Geometry check sheet. Reference: the model listing, model coordinates, mm. Face numbers are marked on the shaded views. A direction names the side the tool comes from. Round coordinates to 2 decimals unless told otherwise and drop trailing zeros. Write each loop counter-clockwise with the first axis right and the second up, starting at its lowest first coordinate (ties: lowest second). Pieces come first, ordered by that corner, then holes. Notation, with made-up numbers: M 11,77.5 L 15,77.5 A26 cw 15,92.5 Z; hole C 57.5,35.5 d3. An arc over 180 degrees is marked long. Answer in a Markdown table with one row per item. Add a question column.
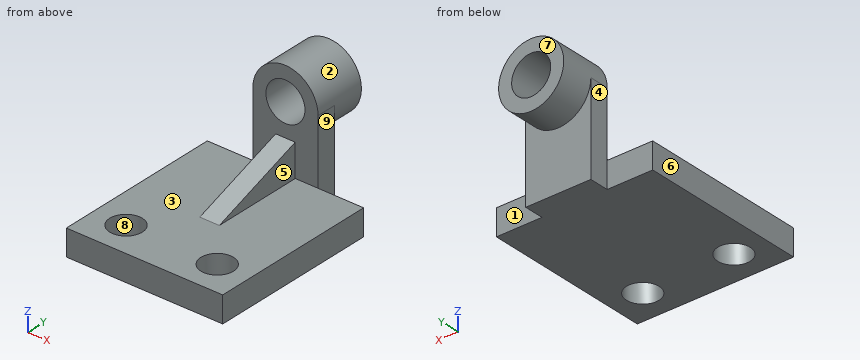
from build123d import *

# Parameters (mm, degrees)
SKETCH_1_W                  = 120
SKETCH_1_H                  = 130
EXTRUDE_1_DEPTH             = 20
SKETCH_2_R                  = 12.5
CUT_EXTRUDE_1_DEPTH         = 91.691785736
SKETCH_3_W                  = 50
SKETCH_3_H                  = 70
EXTRUDE_2_DEPTH             = 15
SKETCH_4_R                  = 25
EXTRUDE_3_DEPTH             = 25
EXTRUDE_3_DIRECTION_2_REACH = 173.828
SKETCH_5_R                  = 15
CUT_EXTRUDE_2_DEPTH         = 204.776838723
RIB_1_REACH                 = 155.786
SKETCH_6_WALL_W             = 383.901473722
SKETCH_6_WALL_H             = 15


with BuildPart() as part:
    # Эскиз1 → Бобышка-Вытянуть1 (new body)
    with BuildSketch(Plane.XY):
        Rectangle(SKETCH_1_W, SKETCH_1_H)
    extrude(amount=EXTRUDE_1_DEPTH)

    # Эскиз2 → Вырез-Вытянуть1 (cut, through all)
    with BuildSketch(Plane.XY.offset(20)):
        with Locations((35, -40)):
            Circle(SKETCH_2_R)
    cut_extrude_1 = extrude(amount=-CUT_EXTRUDE_1_DEPTH, mode=Mode.SUBTRACT)

    # Зеркальное отражение1: Вырез-Вытянуть1 across plane
    add(cut_extrude_1.mirror(Plane(origin=(0, 0, 0), x_dir=(0, 0, 1), z_dir=(1, 0, 0))), mode=Mode.SUBTRACT)

    # Эскиз3 → Бобышка-Вытянуть2 (add)
    with BuildSketch(Plane(origin=(0, 65, 0), x_dir=(1, 0, 0), z_dir=(0, 1, 0))):
        with Locations((0, -35)):
            Rectangle(SKETCH_3_W, SKETCH_3_H)
    extrude(amount=EXTRUDE_2_DEPTH)

    # Эскиз4 → Бобышка-Вытянуть3 (add)
    with BuildSketch(Plane(origin=(0, 80, 0), x_dir=(1, 0, 0), z_dir=(0, 1, 0))):
        with Locations(Location((0, -70, 0), (0, 0, 270))):
            Circle(SKETCH_4_R)
    extrude(amount=EXTRUDE_3_DEPTH)

    # Бобышка-Вытянуть3 direction 2: up to this face of the body (flat: up to its plane)
    extrude_3_direction_2_end = Plane(part.part.faces().sort_by_distance((0, 65, 45))[0])
    # Эскиз4 → Бобышка-Вытянуть3 direction 2 (add, up to the picked face)
    with BuildSketch(Plane(origin=(0, 80, 0), x_dir=(1, 0, 0), z_dir=(0, 1, 0)), mode=Mode.PRIVATE) as extrude_3_direction_2_sk1:
        with Locations(Location((0, -70, 0), (0, 0, 270))):
            Circle(SKETCH_4_R)
    extrude_3_direction_2_tool1 = split(extrude(extrude_3_direction_2_sk1.sketch, amount=-EXTRUDE_3_DIRECTION_2_REACH, mode=Mode.PRIVATE), bisect_by=extrude_3_direction_2_end, keep=Keep.BOTH, mode=Mode.PRIVATE)
    add(extrude_3_direction_2_tool1.solids().sort_by(Axis((0, 80, 70), (0, -1, 0)))[0])

    # Эскиз5 → Вырез-Вытянуть2 (cut, through all)
    with BuildSketch(Plane(origin=(0, 105, 0), x_dir=(1, 0, 0), z_dir=(0, 1, 0))):
        with Locations(Location((0, -70, 0), (0, 0, 270))):
            Circle(SKETCH_5_R)
    extrude(amount=-CUT_EXTRUDE_2_DEPTH, mode=Mode.SUBTRACT)

    # Эскиз6 wall → Ребро1 (add, up to next)
    with BuildSketch(Plane(origin=(0, 30, 32.5), x_dir=(0, -0.941741911595, -0.336336396998), z_dir=(0, 0.336336396998, -0.941741911595)), mode=Mode.PRIVATE) as rib_1_sk1:
        Rectangle(SKETCH_6_WALL_W, SKETCH_6_WALL_H)
    rib_1_tool1 = extrude(rib_1_sk1.sketch, amount=RIB_1_REACH, mode=Mode.PRIVATE) - part.part
    add(rib_1_tool1.solids().sort_by_distance((0, 30, 32.5))[0])


solid = part.part
Item 1: Section check A-A, the plane x = 0. Record the boundary of the cut face in (y, z), and give its area (3 significant figures).
Item 2: Section check D-D, the plane x = -20. Record the boundary of the cut face in (y, z).
Item 3: Scan lines: probe 1 along Y at (x, z) = (-35, 16); probe 2 along X at (y, z) = (96, 70); probe 3 along Y at (x, z) = (4, 13.5). Record each from-to range of solid material in increasing order. Write a range as from..to.
Item 4: Access from +Z, -Z, +X, -X, +Y, -Y to the whole of each face (thin tool, end or side, straight path). Record for the marked faces 1, 2, 3, 4 and 5.
Item 5: Mould release check, pull along X, two halves, no side actions. Record for the marked faces 6, 7, 8 and 9: +X half, -X half, draft (parallel to the pull), parting line (faces both ways), or undercut.
Item 6: Gauge pin test, flat ends, axial feed: pin 1 Ø12 at (y, z) = (74.5, 48.5) entering from -X; pin 2 Ø1 at (y, z) = (6, 22.5) entering from +X; pin 3 Ø16 at (x, z) = (41.5, 13) entering from +Y; pin 4 Ø3 at (x, y) = (-45.5, -25) entering from -Z. Record the tip position at first contact, or that the pin passes through.
Item 7: Section check C-C, the plane z = 28.5. Record the boundary of the cut face in (x, y).
Item 8: Section check B-B, the plane y = 76.5. Record the boundary of the cut face in (x, z), and give its area (3 significant figures).
Result sheet:
| question | item | result |
|---|---|---|
| 1 | outline | M -65,0 L 80,0 L 80,45 L 105,45 L 105,55 L 65,55 L 65,45 L -5,20 L -65,20 Z; M 65,85 L 105,85 L 105,95 L 65,95 Z |
| 1 | area | 4,950 mm^2 |
| 2 | outline | M -65,0 L 80,0 L 80,55 L 105,55 L 105,85 L 65,85 L 65,20 L -65,20 Z |
| 3 | probe 1 | y = -65..-52.5, -27.5..65 |
| 3 | probe 2 | x = -25..-15, 15..25 |
| 3 | probe 3 | y = -65..80 |
| 4 | face 1 | +Z, -Z, +X, +Y |
| 4 | face 2 | +Y |
| 4 | face 3 | +Z, -Y |
| 4 | face 4 | +Z, -Z, -X, +Y |
| 4 | face 5 | +Z, +X, -Y |
| 5 | face 6 | -X half |
| 5 | face 7 | draft |
| 5 | face 8 | undercut |
| 5 | face 9 | +X half |
| 6 | pin 1 | stops at x = -25 |
| 6 | pin 2 | stops at x = 7.5 |
| 6 | pin 3 | stops at y = 65 |
| 6 | pin 4 | stops at z = 0 |
| 7 | outline | M -25,65 L -7.5,65 L -7.5,18.8 L 7.5,18.8 L 7.5,65 L 25,65 L 25,80 L -25,80 Z |
| 8 | outline | M -25,0 L 25,0 L 25,70 A25 ccw -25,70 Z; hole C 0,70 d30 |
| 8 | area | 3,770 mm^2 |
